Geometry check sheet. Reference: the model listing, model coordinates, mm. Face numbers are marked on the shaded views. A direction names the side the tool comes from. Give positions to 0.01 mm unless a question says otherwise; leave off trailing zeros. Loops run counter-clockwise (first coordinate to the right, second up) from the corner with the lowest first, then second, coordinate; pieces in that order, holes last. Notation, with made-up numbers: (50, -15) - (99, -15) arc R18 ccw to (99, -7) - close; hole circle Ø3 at (-21, -29). An arc over 180 degrees is marked (long way). Write item = value, one per line. Start each with the question number.
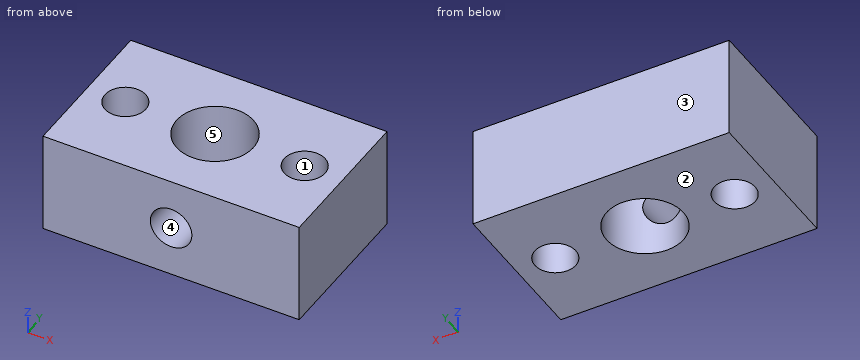
Solid Edge part; units mm, degrees
sketch "Sketch1" plane through (0, 0, 0) normal (0, 0, 1) x (1, 0, 0)
  line L0 (10, -6) -> (-10, -6)
  line L1 (-10, -6) -> (-10, 6)
  line L2 (-10, 6) -> (10, 6)
  line L3 (10, 6) -> (10, -6)
  dimension "D1" = 10
  dimension "D2" = 10
extrude "Protrusion1" add sketch "Sketch1" along normal blind 8
hole "Hole_1" at (0, 0, 8) direction (0, 0, -1) diameter 6 end up to next
hole "Hole_2" at (-7, 0, 8) direction (0, 0, -1) diameter 3.2 end up to next
hole "Hole1" at (7, 0, 8) direction (0, 0, -1) diameter 3.2 end up to next
hole "Hole_4" at (0, -6, 4) direction (0, 1, 0) diameter 3.242 end up to next thread major 4 thread length 2
hole "Hole2" [suppressed]
1) Release check for a two-part mould opening along Y. For the marked faces 1, 2 and 3 record: pulls with the +Y half, pulls with the -Y half, needs draft (parallel to the pull), parting line crosses it, or undercut.
2) Cross-section at A-A on z = 7.25. Enter the section's corners in (x, y).
3) Material ranges on line 1 along X through (y, z) = (0, 6.25); line 2 along Y through (x, z) = (-7, 6.25); line 3 along X through (y, z) = (-0.75, 0.5), recorded low to high.
4) Cross-section at C-C on y = 0. Enter the section's corners in (x, z).
5) Cross-section at B-B on x = 0. Enter the section's corners in (y, z).
6) Tool access check on the marked faces 4 and 5. Record the directions out of +Z, -Z, +X, -X, +Y, -Y that give a thin tool (end or side, any length) a straight path to the whole face; none if there is none.
7) Cross-section at D-D on x = 7. Enter the section's corners in (y, z).
8) Gauge pin test, flat ends, axial feed: P1, Ø4, axis at x = -5, y = -4.5, coming from the -Z side; P2, Ø1.9, axis at x = 0, z = 4, coming from the -Y side; P3, Ø2.5, axis at x = 7, y = 0, coming from the +Z side. Record the tip position at first contact, or that the pin passes through.
Checked values:
q1.face_1 = undercut
q1.face_2 = needs draft
q1.face_3 = pulls with the +Y half
q2.outline = (-10, -6) - (10, -6) - (10, 6) - (-10, 6) - close; hole circle Ø3.2 at (-7, 0); hole circle Ø6 at (0, 0); hole circle Ø3.2 at (7, 0)
q3.line_1 = -10 to -8.6, -5.4 to -3, 3 to 5.4, 8.6 to 10
q3.line_2 = -6 to -1.6, 1.6 to 6
q3.line_3 = -10 to -8.41, -5.59 to -2.9, 2.9 to 5.59, 8.41 to 10
q4.outline = (-10, 0) - (-8.6, 0) - (-8.6, 8) - (-10, 8) - close; (-5.4, 0) - (-3, 0) - (-3, 8) - (-5.4, 8) - close; (3, 0) - (5.4, 0) - (5.4, 8) - (3, 8) - close; (8.6, 0) - (10, 0) - (10, 8) - (8.6, 8) - close
q5.outline = (-6, 0) - (-3, 0) - (-3, 2.38) - (-6, 2.38) - close; (-6, 5.62) - (-3, 5.62) - (-3, 8) - (-6, 8) - close; (3, 0) - (6, 0) - (6, 8) - (3, 8) - close
q6.face_4 = -Y
q6.face_5 = +Z, -Z
q7.outline = (-6, 0) - (-1.6, 0) - (-1.6, 8) - (-6, 8) - close; (1.6, 0) - (6, 0) - (6, 8) - (1.6, 8) - close
q8.P1 = 0
q8.P2 = 2.85
q8.P3 = through
